from build123d import *

# Parameters (mm, degrees)
SKETCH1_W               = 70
SKETCH1_H               = 40
BOSS_EXTRUDE1_DEPTH     = 10
BOSS_EXTRUDE2_DEPTH     = 30
CUT_EXTRUDE1_DEPTH      = 57.789083458
CUT_EXTRUDE1_DEPTH_BACK = 57.789083458
SKETCH3_OUTSIDE_W       = 90
SKETCH3_OUTSIDE_H       = 60


with BuildPart() as part:
    # Sketch1 → Boss-Extrude1 (new body)
    with BuildSketch(Plane(origin=(0, 0, 0), x_dir=(1, 0, 0), z_dir=(0, 1, 0))):
        Rectangle(SKETCH1_W, SKETCH1_H)
    extrude(amount=BOSS_EXTRUDE1_DEPTH)

    # Sketch2 → Boss-Extrude2 (add)
    with BuildSketch(Plane(origin=(0, 10, 0), x_dir=(1, 0, 0), z_dir=(0, 1, 0))):
        Polygon((-35, 20), (-35, 0), (4.372843299, 0), (14.372843299, 10), (35, 10), (35, 20), align=None)
    extrude(amount=BOSS_EXTRUDE2_DEPTH)

    # Sketch3 outside → Cut-Extrude1 (cut, two sides: drawn at the far end of the back side and taken through both)
    with BuildSketch(Plane.XY.offset(-CUT_EXTRUDE1_DEPTH_BACK)):
        with Locations((0, 20)):
            Rectangle(SKETCH3_OUTSIDE_W, SKETCH3_OUTSIDE_H)
        with BuildLine():
            Line((-25.31357835, 40), (-35, 40))
            Line((-35, 40), (-35, 0))
            Line((-35, 0), (35, 0))
            Line((35, 0), (35, 10))
            Line((35, 10), (14.372843299, 40))
            Line((14.372843299, 40), (-5.31357835, 40))
            ThreePointArc((-5.31357835, 40), (-15.31357835, 30), (-25.31357835, 40))
        make_face(mode=Mode.SUBTRACT)
    extrude(amount=CUT_EXTRUDE1_DEPTH + CUT_EXTRUDE1_DEPTH_BACK, mode=Mode.SUBTRACT)


solid = part.part
Geometry check sheet. Reference: the model listing, model coordinates, mm. A direction names the side the tool comes from. Give positions to 0.01 mm unless a question says otherwise; leave off trailing zeros. Loops run counter-clockwise (first coordinate to the right, second up) from the corner with the lowest first, then second, coordinate; pieces in that order, holes last.
(1) Section check D-D on y = 24.5. Record the cut outline in (x, z), then the cut area to 3 significant figures.
From the geometry:
outline: (-35, -20) - (25.03, -20) - (25.03, -10) - (14.37, -10) - (4.37, 0) - (-35, 0) - close
area: 1,040 mm2
(2) Depth check by flat-ended pin: pin 1 Ø8 at (x, y) = (-16.5, 29.5) entering from +Z. Enter the tip coordinate at first touch or a pass-through.
From the geometry:
pin 1: stops at z = 0
(3) Release check for a two-part mould opening along X. For faces 4 (the flat face through (0, 5, 20)), 5 (the flat face through (9.303, 24.79, -4.93)), 6 (the cylindrical face through (-15.094, 30.002, -10.14)) record: released by +X, released by -X, zero draft, split by the parting line, or undercut.
From the geometry:
face 4: zero draft
face 5: released by +X
face 6: undercut
(4) Section check C-C on x = 1. Record the cut outline in (y, z), then the cut area to 3 significant figures.
From the geometry:
outline: (0, -20) - (40, -20) - (40, 0) - (10, 0) - (10, 20) - (0, 20) - close
area: 1,000 mm2
(5) Section check B-B on z = -14.5. Record the cut outline in (x, y), then the cut area to 3 significant figures.
From the geometry:
outline: (-35, 0) - (35, 0) - (35, 10) - (14.37, 40) - (-5.31, 40) arc R10 cw to (-25.31, 40) - (-35, 40) - close
area: 2,330 mm2
(6) Section check A-A on y = 32.5. Record the cut outline in (x, z), then the cut area to 3 significant figures.
From the geometry:
outline: (-35, -20) - (-21.93, -20) - (-21.93, 0) - (-35, 0) - close; (-8.7, -20) - (19.53, -20) - (19.53, -10) - (14.37, -10) - (4.37, 0) - (-8.7, 0) - close
area: 724 mm2
(7) Set-up check for faces 1 (the flat face through (-16, 21, 0)), 2 (the flat face through (-35, 15, -5)), 3 (the flat face through (22, 21, -10)): record each of +Z, -Z, +X, -X, +Y, -Y from which the full face is reachable in a straight line by a thin tool's end or side.
From the geometry:
face 1: +Z, +X, -X, +Y
face 2: +Z, -Z, -X, +Y, -Y
face 3: +Z, +X, +Y
(8) Thickness scan on L1, parallel to Y at x = -21, z = 13.5; L2, parallel to Z at x = -30, y = 20; L3, parallel to X at y = 36, z = -1. Record the ranges inside material, lowest first.
From the geometry:
L1: y = 0 to 10
L2: z = -20 to 0
L3: x = -35 to -24.48, -6.15 to 5.37
